For this review, use the dimensioned drawing (mm, ordinates from the lowest corner) and the shaded views. Coordinates: 2 decimals unless noted, no trailing zeros. Write each loop counter-clockwise with the first axis right and the second up, starting at its lowest first coordinate (ties: lowest second). Pieces come first, ordered by that corner, then holes.
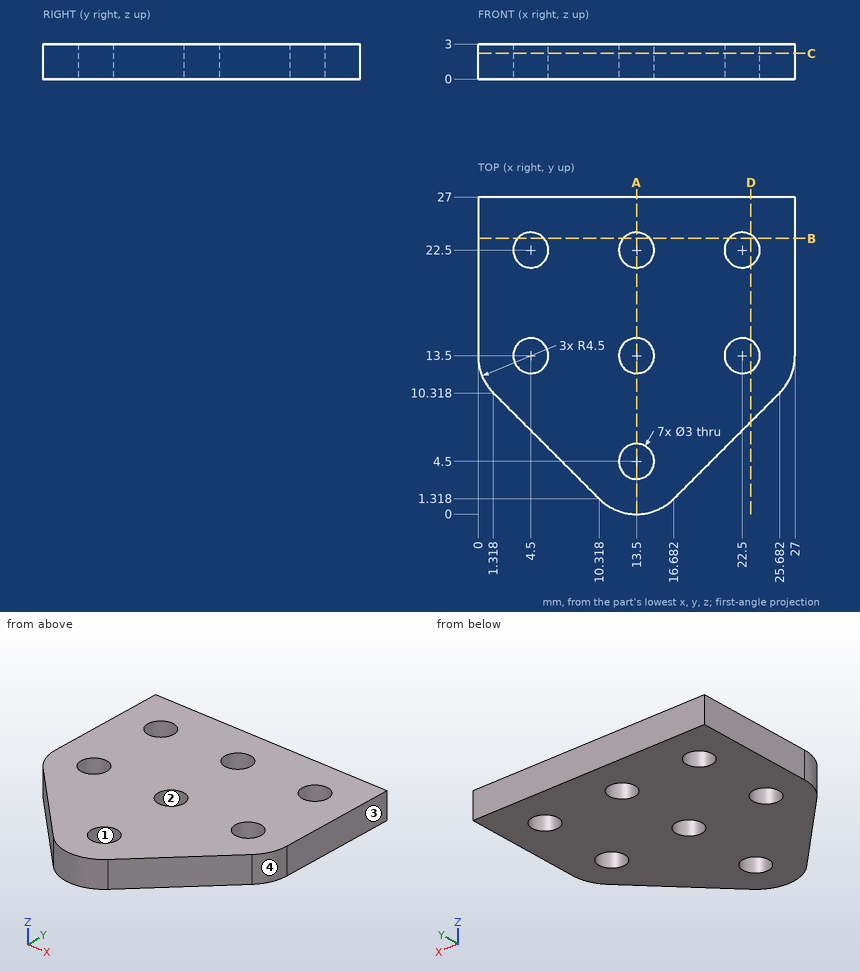
(1) Consider section A-A (x = 13.5). Give the boundary of the cut face in (y, z).
(2) Consider section D-D (x = 23.25). Give the boundary of the cut face in (y, z).
(3) Consider section C-C (z = 2.2). Give the boundary of the cut face in (x, y), plus the area to 3 significant figures.
(4) Insertion check: pin 1 Ø1.5 at (x, z) = (17.5, 1) entering from -Y. The pin has a flat end and moves straight along its axis. Give the tip position at first contact, or say it passes through.
(5) Mouldability with a two-part tool opening along Y and no side actions: class the marked faces 1, 2, 3 and 4 as +Y half, -Y half, draft (parallel to the pull), parting line (faces both ways), or undercut.
(6) Wall thickness on line 1 (X direction, y = 22.5, z = 1.45); line 2 (X direction, y = 14.75, z = 1.4): over which ranges is each line inside the solid? List them lowest first.
(7) Consider section B-B (y = 23.5). Give the boundary of the cut face in (x, z).
Results:
1. outline: (0, 0) - (3, 0) - (3, 3) - (0, 3) - close; (6, 0) - (12, 0) - (12, 3) - (6, 3) - close; (15, 0) - (21, 0) - (21, 3) - (15, 3) - close; (24, 0) - (27, 0) - (27, 3) - (24, 3) - close
2. outline: (7.89, 0) - (12.2, 0) - (12.2, 3) - (7.89, 3) - close; (14.8, 0) - (21.2, 0) - (21.2, 3) - (14.8, 3) - close; (23.8, 0) - (27, 0) - (27, 3) - (23.8, 3) - close
3. outline: (0, 13.5) arc R4.5 ccw to (1.32, 10.32) - (10.32, 1.32) arc R4.5 ccw to (16.68, 1.32) - (25.68, 10.32) arc R4.5 ccw to (27, 13.5) - (27, 27) - (0, 27) - close; hole circle Ø3 at (4.5, 13.5); hole circle Ø3 at (4.5, 22.5); hole circle Ø3 at (13.5, 4.5); hole circle Ø3 at (13.5, 13.5); hole circle Ø3 at (13.5, 22.5); hole circle Ø3 at (22.5, 13.5); hole circle Ø3 at (22.5, 22.5)
3. area: 542 mm2
4. pin 1: stops at y = 1.39
5. face 1: undercut
5. face 2: undercut
5. face 3: draft
5. face 4: -Y half
6. line 1: x = 0 to 3, 6 to 12, 15 to 21, 24 to 27
6. line 2: x = 0 to 3.67, 5.33 to 12.67, 14.33 to 21.67, 23.33 to 27
7. outline: (0, 0) - (3.38, 0) - (3.38, 3) - (0, 3) - close; (5.62, 0) - (12.38, 0) - (12.38, 3) - (5.62, 3) - close; (14.62, 0) - (21.38, 0) - (21.38, 3) - (14.62, 3) - close; (23.62, 0) - (27, 0) - (27, 3) - (23.62, 3) - close
